Source: CAD feature listing. Evaluate the final solid. Frame: model axes, mm. Face numbers are marked on the shaded views. Coordinates: 2 decimals unless noted, no trailing zeros. Loops run counter-clockwise (first coordinate to the right, second up) from the corner with the lowest first, then second, coordinate; pieces in that order, holes last. Notation, with made-up numbers: (61.25, 88) -> (104.25, 88) arc R30 cw to (104.25, 116) -> close; hole circle Ø11 at (1, 19.25). An arc over 180 degrees is marked (long way). Answer as CSV lines item,"result".
from build123d import *

# Parameters (mm, degrees)
F1_DEPTH = 95
F2_DEPTH = 93.7


with BuildPart() as f1:
    # F0 (on Top) → F1 (new body)
    with BuildSketch(Plane.XY):
        with BuildLine():
            Line((7.6, -21.177582), (7.6, -23.816801))
            ThreePointArc((7.6, -23.816801), (25, 0), (7.6, 23.816801))
            Line((7.6, 23.816801), (7.6, 21.177582))
            Line((7.6, 21.177582), (7.6, -21.177582))
        make_face()
        with BuildLine():
            ThreePointArc((8.8, 22.113344), (23.8, 0), (8.8, -22.113344))
            Line((8.8, -22.113344), (8.8, 22.113344))
        make_face(mode=Mode.SUBTRACT)
    extrude(amount=F1_DEPTH)

    # F0 (on Top) → F2 (join)
    with BuildSketch(Plane.XY):
        with BuildLine():
            Line((8.8, 22.113344), (8.8, -22.113344))
            ThreePointArc((8.8, -22.113344), (23.8, 0), (8.8, 22.113344))
        make_face()
        with BuildLine():
            ThreePointArc((10.1, 20.105721), (22.5, 0), (10.1, -20.105721))
            Line((10.1, -20.105721), (10.1, 20.105721))
        make_face(mode=Mode.SUBTRACT)
    extrude(amount=F2_DEPTH)


solid = f1.part
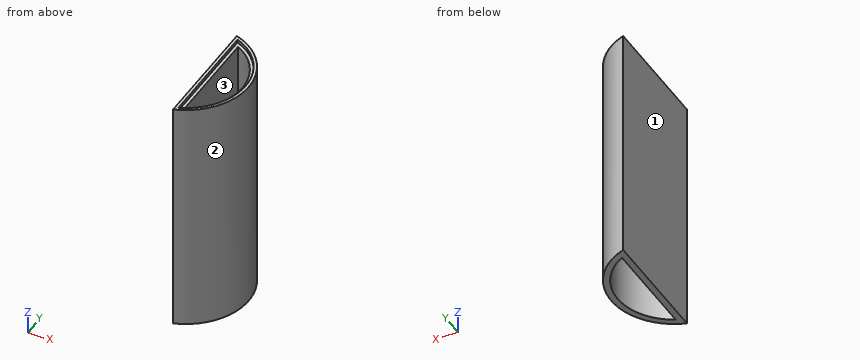
(1) Cut plane B-B (x = 16.5). Return the cut outline in (y, z).
Computed values:
outline,"(-18.78, 0) -> (-15.3, 0) -> (-15.3, 93.7) -> (-17.15, 93.7) -> (-17.15, 95) -> (-18.78, 95) -> close; (15.3, 0) -> (18.78, 0) -> (18.78, 95) -> (17.15, 95) -> (17.15, 93.7) -> (15.3, 93.7) -> close"
(2) Material intervals for L1, parallel to X at y = 0, z = 53.5; L2, parallel to Z at x = 19.25, y = -12; L3, parallel to Y at x = 18.5, z = 38, sorted ascending. Write a range as [from, to].
Computed values:
L1,"[7.6, 10.1], [22.5, 25]"
L2,"[0, 93.7]"
L3,"[-16.82, -12.81], [12.81, 16.82]"
(3) Cut plane A-A (y = 0). Return the cut outline in (x, z).
Computed values:
outline,"(7.6, 0) -> (10.1, 0) -> (10.1, 93.7) -> (8.8, 93.7) -> (8.8, 95) -> (7.6, 95) -> close; (22.5, 0) -> (25, 0) -> (25, 95) -> (23.8, 95) -> (23.8, 93.7) -> (22.5, 93.7) -> close"
(4) Draft query along X for the marked faces 1, 2 and 3. Return one class per face: released by +X, released by -X, zero draft, split by the parting line, or undercut.
Computed values:
face 1,"released by -X"
face 2,"released by +X"
face 3,"undercut"
(5) Pin query (flat end, axial travel): pin 1 Ø1 at (x, z) = (9.5, 20.5) entering from +Y; pin 2 Ø1 at (y, z) = (-7.5, 46.5) entering from +X; pin 3 Ø4 at (y, z) = (-14.5, 27.5) entering from +X. Return the tip coordinate at first contact, or that it passes through.
Computed values:
pin 1,"y = 23.32"
pin 2,"x = 24"
pin 3,"x = 21.65"
(6) Cut plane C-C (z = 73). Return the cut outline in (x, y), then the cut area to 3 significant figures.
Computed values:
outline,"(7.6, -23.82) arc R25 ccw to (7.6, 23.82) -> close; hole (10.1, -20.11) arc R22.5 ccw to (10.1, 20.11) -> close"
area,"251 mm^2"
